Source: CAD feature listing. Evaluate the final solid. Frame: model axes, mm. A direction names the side the tool comes from. Give positions to 0.01 mm unless a question says otherwise; leave off trailing zeros. Loops run counter-clockwise (first coordinate to the right, second up) from the corner with the lowest first, then second, coordinate; pieces in that order, holes last.
```python
from build123d import *

# Parameters (mm, degrees)
F0_W     = 112
F0_H     = 77
F1_DEPTH = 3
F2_W     = 8
F2_H     = 8
F3_DEPTH = 4
F4_R     = 2
F5_DEPTH = 25.4
F6_R     = 3.1
F6_R_2   = 2
F7_DEPTH = 5


with BuildPart() as f1:
    # F0 (on Top) → F1 (new body)
    with BuildSketch(Plane.XY):
        Rectangle(F0_W, F0_H)
    extrude(amount=F1_DEPTH)

    # F2 (on face) → F3 (join)
    with BuildSketch(Plane.XY.offset(3)):
        with Locations((-52, 34.5)):
            Rectangle(F2_W, F2_H)
        with Locations((-52, -34.5)):
            Rectangle(F2_W, F2_H)
        with Locations((52, -34.5)):
            Rectangle(F2_W, F2_H)
        with Locations((52, 34.5)):
            Rectangle(F2_W, F2_H)
    extrude(amount=F3_DEPTH)

    # F4 (on face) → F5 (cut)
    with BuildSketch(Plane.XY.offset(7)):
        with Locations((-52, 34.5)):
            Circle(F4_R)
        with Locations((52, 34.5)):
            Circle(F4_R)
        with Locations((-52, -34.5)):
            Circle(F4_R)
        with Locations((52, -34.5)):
            Circle(F4_R)
    extrude(amount=-F5_DEPTH, mode=Mode.SUBTRACT)

    # F6 (on face) → F7 (cut)
    with BuildSketch(Plane(origin=(0, 0, 0), x_dir=(1, 0, 0), z_dir=(0, 0, -1))):
        with Locations((-52, 34.5)):
            Circle(F6_R)
        with Locations((-52, 34.5)):
            Circle(F6_R_2, mode=Mode.SUBTRACT)
        with Locations((52, 34.5)):
            Circle(F6_R)
        with Locations((52, 34.5)):
            Circle(F6_R_2, mode=Mode.SUBTRACT)
        with Locations((52, -34.5)):
            Circle(F6_R)
        with Locations((52, -34.5)):
            Circle(F6_R_2, mode=Mode.SUBTRACT)
        with Locations((-52, -34.5)):
            Circle(F6_R)
        with Locations((-52, -34.5)):
            Circle(F6_R_2, mode=Mode.SUBTRACT)
    extrude(amount=-F7_DEPTH, mode=Mode.SUBTRACT)


solid = f1.part
```
(1) First-contact query: pin 1 (1.5 mm diameter, centred on x = -11.5, y = -4.5, fed in from +Z); pin 2 (3 mm diameter, centred on x = 53, y = -33.5, fed in from -Z). Flat tips, straight axial feed; report the tip coordinate or a pass-through.
A:
pin 1: stops at z = 3
pin 2: stops at z = 5
(2) Section A-A, the plane x = -52. Return the cut outline in (y, z).
A:
outline: (-38.5, 0) - (-37.6, 0) - (-37.6, 5) - (-36.5, 5) - (-36.5, 7) - (-38.5, 7) - close; (-32.5, 5) - (-31.4, 5) - (-31.4, 0) - (31.4, 0) - (31.4, 5) - (32.5, 5) - (32.5, 7) - (30.5, 7) - (30.5, 3) - (-30.5, 3) - (-30.5, 7) - (-32.5, 7) - close; (36.5, 5) - (37.6, 5) - (37.6, 0) - (38.5, 0) - (38.5, 7) - (36.5, 7) - close
(3) Section B-B, the plane y = -34.5. Return the cut outline in (x, z).
A:
outline: (-56, 0) - (-55.1, 0) - (-55.1, 5) - (-54, 5) - (-54, 7) - (-56, 7) - close; (-50, 5) - (-48.9, 5) - (-48.9, 0) - (48.9, 0) - (48.9, 5) - (50, 5) - (50, 7) - (48, 7) - (48, 3) - (-48, 3) - (-48, 7) - (-50, 7) - close; (54, 5) - (55.1, 5) - (55.1, 0) - (56, 0) - (56, 7) - (54, 7) - close
(4) Reachability of faces 5 (the flat face through (-1, 1, 3)), 6 (the flat face through (48, -35, 5)), 7 (the flat face through (52, -32, 5)) from +Z, -Z, +X, -X, +Y, -Y: full face, straight path, thin tool, end or side. Return the list, or none.
A:
face 5: +Z
face 6: +Z, +Y, -Y
face 7: -Z
(5) Section C-C, the plane x = 24.5. Return the cut outline in (y, z).
A:
outline: (-38.5, 0) - (38.5, 0) - (38.5, 3) - (-38.5, 3) - close
(6) Mould query, pull axis Y, two halves, no side actions, for faces 1 (the flat face through (-1, 38.5, 2)), 2 (the flat face through (-1, 1, 0)), 3 (the cylindrical face through (53.67, -37.11, 2.46)), 4 (the cylindrical face through (53.67, 31.89, 2.46)). Classes: pulls with the +Y half, pulls with the -Y half, needs draft (parallel to the pull), parting line crosses it, or undercut.
A:
face 1: pulls with the +Y half
face 2: needs draft
face 3: undercut
face 4: undercut
(7) Ray query, line 1 along Y through (x, z) = (-52, 6.4); line 2 along X through (y, z) = (34.5, 6.3); line 3 along X through (y, z) = (-34.5, 3.7). Return the intervals inside material, ascending.
A:
line 1: y = -38.5 to -36.5, -32.5 to -30.5, 30.5 to 32.5, 36.5 to 38.5
line 2: x = -56 to -54, -50 to -48, 48 to 50, 54 to 56
line 3: x = -56 to -55.1, -48.9 to -48, 48 to 48.9, 55.1 to 56
(8) Section D-D, the plane y = 2.5. Return the cut outline in (x, z).
A:
outline: (-56, 0) - (56, 0) - (56, 3) - (-56, 3) - close
